```python
from build123d import *

# Parameters (mm, degrees)
SKETCH1_W            = 54.99
SKETCH1_H            = 54.99
BOSS_EXTRUDE1_DEPTH  = 6
M3_CLEARANCE_HOLE2_D = 3.4
SKETCH8_W            = 10.18
SKETCH8_H            = 18.5
BOSS_EXTRUDE2_DEPTH  = 11


with BuildPart() as part:
    # Sketch1 → Boss-Extrude1 (new body)
    with BuildSketch(Plane(origin=(0, 0, 0), x_dir=(1, 0, 0), z_dir=(0, 1, 0))):
        Rectangle(SKETCH1_W, SKETCH1_H)
    extrude(amount=BOSS_EXTRUDE1_DEPTH)

    # M3 Clearance Hole2 (through all)
    with Locations(Plane(origin=(0, 6, 0), x_dir=(1, 0, 0), z_dir=(0, 1, 0))):
        with Locations((-24.095, 24.095), (24.095, 24.095), (24.095, -24.095), (-24.095, -24.095)):
            Hole(M3_CLEARANCE_HOLE2_D / 2)

    # Sketch8 → Boss-Extrude2 (add)
    with BuildSketch(Plane(origin=(0, 6, 0), x_dir=(1, 0, 0), z_dir=(0, 1, 0))):
        with Locations((-11.325, 26.245)):
            Rectangle(SKETCH8_W, SKETCH8_H)
        with Locations((10.605, 26.245)):
            Rectangle(SKETCH8_W, SKETCH8_H)
        with Locations((15.405, -26.245)):
            Rectangle(SKETCH8_W, SKETCH8_H)
    extrude(amount=BOSS_EXTRUDE2_DEPTH)


solid = part.part
```
Geometry: final body of the model. Coordinates: model frame, mm. A direction names the side the tool comes from. Round coordinates to 2 decimals unless told otherwise and drop trailing zeros. Loops run counter-clockwise (first coordinate to the right, second up) from the corner with the lowest first, then second, coordinate; pieces in that order, holes last.
Item 1: Line query: L1, parallel to X at y = 5, z = 25 (3 decimals); L2, parallel to X at y = 15.75, z = -31.5 (3 decimals); L3, parallel to Z at x = -23.5, y = 5.75 (3 decimals). Output: solid intervals per line, ascending.
Checked values:
L1: x = -27.495 to -25.534, -22.656 to 22.656, 25.534 to 27.495
L2: x = -16.415 to -6.235, 5.515 to 15.695
L3: z = -27.495 to -25.687, -22.503 to 22.503, 25.687 to 27.495
Item 2: Reachability of faces 4 (the flat face through (5.515, 11, -26)), 5 (the flat face through (0, 3, -27.495)), 6 (the flat face through (-11, 11, -16.995)), 7 (the flat face through (11, 11, -16.995)), 8 (the flat face through (-16.415, 11, -26)) from +Z, -Z, +X, -X, +Y, -Y: full face, straight path, thin tool, end or side. Return the list, or none.
Checked values:
face 4: +Z, -Z, +Y
face 5: -Z, +X, -X, -Y
face 6: +Z, +X, -X, +Y
face 7: +X, -X, +Y
face 8: +Z, -Z, -X, +Y
Item 3: Section C-C, the plane x = 8.5. Output: boundary loops of the cut face in (y, z) (3 decimals).
Checked values:
outline: (0, -27.495) - (6, -27.495) - (6, -35.495) - (17, -35.495) - (17, -16.995) - (6, -16.995) - (6, 27.495) - (0, 27.495) - close
Item 4: Section A-A, the plane y = 9.75. Output: boundary loops of the cut face in (x, z) (3 decimals).
Checked values:
outline: (-16.415, -35.495) - (-6.235, -35.495) - (-6.235, -16.995) - (-16.415, -16.995) - close; (5.515, -35.495) - (15.695, -35.495) - (15.695, -16.995) - (5.515, -16.995) - close; (10.315, 16.995) - (20.495, 16.995) - (20.495, 35.495) - (10.315, 35.495) - close
Item 5: Section B-B, the plane z = -21.5. Output: boundary loops of the cut face in (x, y) (3 decimals).
Checked values:
outline: (-27.495, 0) - (27.495, 0) - (27.495, 6) - (15.695, 6) - (15.695, 17) - (5.515, 17) - (5.515, 6) - (-6.235, 6) - (-6.235, 17) - (-16.415, 17) - (-16.415, 6) - (-27.495, 6) - close
Item 6: Mould query, pull axis Z, two halves, no side actions, for faces 1 (the flat face through (0, 3, 27.495)), 2 (the flat face through (20.495, 11, 26)), 3 (the cylindrical face through (-25.01, 2.96, -25.53)). Classes: released by +Z, released by -Z, zero draft, split by the parting line, or undercut.
Checked values:
face 1: released by +Z
face 2: zero draft
face 3: undercut
Item 7: Contact query for flat-ended pins moving along their axis: P1, Ø3, axis at x = -11, y = 11.5, coming from the +Z side (3 decimals); P2, Ø4, axis at x = 15.5, z = 33.5, coming from the -Y side; P3, Ø4.5, axis at x = 24.095, z = 24.095, coming from the -Y side; P4, Ø9, axis at y = 13, z = -24.5, coming from the +X side (3 decimals). Output: stop coordinate, or through.
Checked values:
P1: stops at z = -16.995
P2: stops at y = 6
P3: stops at y = 0
P4: stops at x = 15.695
Item 8: Section D-D, the plane z = 19.5. Output: boundary loops of the cut face in (x, y) (3 decimals).
Checked values:
outline: (-27.495, 0) - (27.495, 0) - (27.495, 6) - (20.495, 6) - (20.495, 17) - (10.315, 17) - (10.315, 6) - (-27.495, 6) - close
